Check sheet for the modelled part. Datum: model origin and axes. Units: mm. A direction names the side the tool comes from. Give positions to 0.01 mm unless a question says otherwise; leave off trailing zeros. Write each loop counter-clockwise with the first axis right and the second up, starting at its lowest first coordinate (ties: lowest second). Pieces come first, ordered by that corner, then holes.
from build123d import *

# Parameters (mm, degrees)
SKETCH1_W           = 11.176
SKETCH1_H           = 3.048
SKETCH1_W_2         = 20.574
SKETCH1_H_2         = 7.62
SKETCH1_W_3         = 23.7998
SKETCH1_H_3         = 12.7
SKETCH1_R           = 1.5875
BOSS_EXTRUDE1_DEPTH = 1.6764
SKETCH1_3_W         = 23.7998
SKETCH1_3_H         = 12.7
BOSS_EXTRUDE2_DEPTH = 10.414
SKETCH1_4_W         = 20.574
SKETCH1_4_H         = 7.62
BOSS_EXTRUDE3_DEPTH = 11.811
SKETCH1_5_W         = 11.176
SKETCH1_5_H         = 3.048
BOSS_EXTRUDE4_DEPTH = 25.4


with BuildPart() as part:
    # Sketch1 → Boss-Extrude1 (new body)
    with BuildSketch(Plane(origin=(0, 0, 0), x_dir=(1, 0, 0), z_dir=(0, 1, 0))):
        with Locations((0, -12.827)):
            Rectangle(SKETCH1_W, SKETCH1_H)
        with Locations((0, -4.445)):
            Rectangle(SKETCH1_W_2, SKETCH1_H_2)
        with Locations((0, 10.287)):
            Rectangle(SKETCH1_W_3, SKETCH1_H_3)
        with BuildLine():
            ThreePointArc((-17.145, 14.351), (-16.401051224, 16.147051224), (-14.605, 16.891))
            Line((-14.605, 16.891), (14.605, 16.891))
            ThreePointArc((14.605, 16.891), (16.401051224, 16.147051224), (17.145, 14.351))
            Line((17.145, 14.351), (17.145, -14.351))
            ThreePointArc((17.145, -14.351), (16.401051224, -16.147051224), (14.605, -16.891))
            Line((14.605, -16.891), (-14.605, -16.891))
            ThreePointArc((-14.605, -16.891), (-16.401051224, -16.147051224), (-17.145, -14.351))
            Line((-17.145, -14.351), (-17.145, 14.351))
        make_face()
        with Locations((14.605, 14.351)):
            Circle(SKETCH1_R, mode=Mode.SUBTRACT)
        with Locations((12.573, -14.351)):
            Circle(SKETCH1_R, mode=Mode.SUBTRACT)
        with Locations((-12.573, -14.351)):
            Circle(SKETCH1_R, mode=Mode.SUBTRACT)
        with Locations((-14.605, 14.351)):
            Circle(SKETCH1_R, mode=Mode.SUBTRACT)
        with Locations((0, -12.827)):
            Rectangle(SKETCH1_W, SKETCH1_H, mode=Mode.SUBTRACT)
        with Locations((0, -4.445)):
            Rectangle(SKETCH1_W_2, SKETCH1_H_2, mode=Mode.SUBTRACT)
        with Locations((0, 10.287)):
            Rectangle(SKETCH1_W_3, SKETCH1_H_3, mode=Mode.SUBTRACT)
    extrude(amount=BOSS_EXTRUDE1_DEPTH)

    # Sketch1_3 → Boss-Extrude2 (add)
    with BuildSketch(Plane(origin=(0, 0, 0), x_dir=(1, 0, 0), z_dir=(0, 1, 0))):
        with Locations((0, 10.287)):
            Rectangle(SKETCH1_3_W, SKETCH1_3_H)
    extrude(amount=BOSS_EXTRUDE2_DEPTH)

    # Sketch1_4 → Boss-Extrude3 (add)
    with BuildSketch(Plane(origin=(0, 0, 0), x_dir=(1, 0, 0), z_dir=(0, 1, 0))):
        with Locations((0, -4.445)):
            Rectangle(SKETCH1_4_W, SKETCH1_4_H)
    extrude(amount=BOSS_EXTRUDE3_DEPTH)

    # Sketch1_5 → Boss-Extrude4 (add)
    with BuildSketch(Plane(origin=(0, 0, 0), x_dir=(1, 0, 0), z_dir=(0, 1, 0))):
        with Locations((0, -12.827)):
            Rectangle(SKETCH1_5_W, SKETCH1_5_H)
    extrude(amount=BOSS_EXTRUDE4_DEPTH)


solid = part.part
1) Sectioned sample at C-C on x = 13.5. Record the boundary of the cut face in (y, z), then the cut area to 3 significant figures.
2) Sectioned sample at B-B on x = -12.5. Record the boundary of the cut face in (y, z), then the cut area to 3 significant figures.
3) Draft check along Z on faces 5 (the flat face through (0, 6, -3.937)), 6 (the cylindrical face through (16.38, 0.83, -16.17)), 7 (the flat face through (0, 10.414, -10)). Enter one of: +Z half, -Z half, draft (parallel to the pull), parting line (faces both ways), or undercut.
4) Sectioned sample at A-A on y = 9.75. Record the boundary of the cut face in (x, z) (3 decimals), then the cut area to 3 significant figures.
5) Scan lines: L1, parallel to Z at x = 0, y = 9 (3 decimals); L2, parallel to Z at x = 8.5, y = 4 (3 decimals); L3, parallel to Z at x = 1, y = 22.5. Record each from-to range of solid material in increasing order.
6) Gauge pin test, flat ends, axial feed: pin 1 (1.9 mm diameter, centred on x = 12.573, z = 14.351, fed in from +Y); pin 2 (8 mm diameter, centred on x = -10, z = -2.5, fed in from +Y); pin 3 (1 mm diameter, centred on x = -5.5, y = 19, fed in from +Z); pin 4 (4.5 mm diameter, centred on x = -5.5, y = 4.5, fed in from -Z). Record the tip position at first contact, or that the pin passes through.
7) Access from +Z, -Z, +X, -X, +Y, -Y to the whole of each face (thin tool, end or side, straight path). Record for faces 1 (the flat face through (0, 11.811, 4)), 2 (the flat face through (-5.588, 13, 13)), 3 (the flat face through (5.588, 13, 13)), 4 (the flat face through (0, 7, 0.635)).
8) Sectioned sample at D-D on x = 9. Record the boundary of the cut face in (y, z) (3 decimals).
Answers below:
1. outline: (0, -16.89) - (1.68, -16.89) - (1.68, -15.49) - (0, -15.49) - close; (0, -13.21) - (1.68, -13.21) - (1.68, 13.06) - (0, 13.06) - close; (0, 15.64) - (1.68, 15.64) - (1.68, 16.89) - (0, 16.89) - close
1. area: 48.5 mm2
2. outline: (0, -16.89) - (1.68, -16.89) - (1.68, 12.77) - (0, 12.77) - close; (0, 15.94) - (1.68, 15.94) - (1.68, 16.89) - (0, 16.89) - close
2. area: 51.3 mm2
3. face 5: undercut
3. face 6: -Z half
3. face 7: draft
4. outline: (-11.9, -16.637) - (11.9, -16.637) - (11.9, -3.937) - (-11.9, -3.937) - close; (-10.287, 0.635) - (10.287, 0.635) - (10.287, 8.255) - (-10.287, 8.255) - close; (-5.588, 11.303) - (5.588, 11.303) - (5.588, 14.351) - (-5.588, 14.351) - close
4. area: 493 mm2
5. L1: z = -16.637 to -3.937, 0.635 to 8.255, 11.303 to 14.351
5. L2: z = -16.637 to -3.937, 0.635 to 8.255
5. L3: z = 11.3 to 14.35
6. pin 1: passes through
6. pin 2: stops at y = 11.81
6. pin 3: stops at z = 14.35
6. pin 4: stops at z = -16.64
7. face 1: -Z, +X, -X, +Y
7. face 2: +Z, -X, +Y
7. face 3: +Z, +X, +Y
7. face 4: +X, -X, +Y
8. outline: (0, -16.891) - (1.676, -16.891) - (1.676, -16.637) - (10.414, -16.637) - (10.414, -3.937) - (1.676, -3.937) - (1.676, 0.635) - (11.811, 0.635) - (11.811, 8.255) - (1.676, 8.255) - (1.676, 16.891) - (0, 16.891) - close
